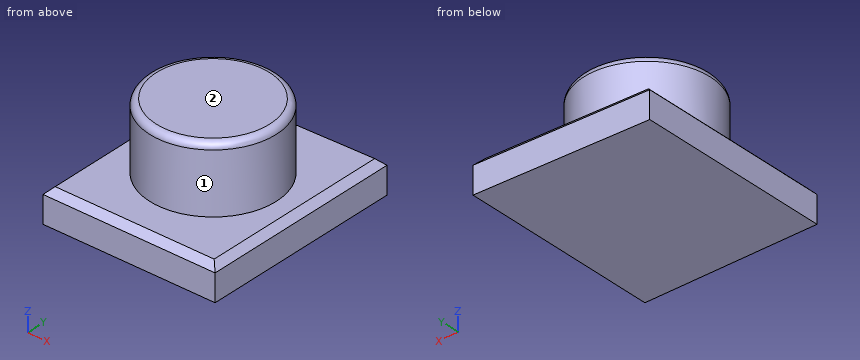
```python
from build123d import *

# Parameters (mm, degrees)
F1_DEPTH = 25.4
F2_R     = 48.0357441032
F3_DEPTH = 50.8
F4_R     = 5
F5_SIZE  = 5


# Not quite as in the source:
# - the program builds the solid bodies; features that only make, move or delete a surface that nothing else refers to are left out


with BuildPart() as f1:
    # F0 (on Top) → F1 (new body)
    with BuildSketch(Plane.XY):
        Polygon((118.1704625487, 0), (-12.6199126244, -4.1209459305), (-12.6199126244, -153.0908346176), (118.1704625487, -153.0908346176), align=None)
    extrude(amount=F1_DEPTH)

    # F2 (on face) → F3 (join)
    with BuildSketch(Plane.XY.offset(25.4)):
        with Locations((51.9535280764, -77.3641169071)):
            Circle(F2_R)
    extrude(amount=F3_DEPTH)

    # F4
    f4_edges = [f1.edges().sort_by_distance(p)[0] for p in [
        (3.917784, -77.364117, 76.2),
    ]]
    fillet(f4_edges, radius=F4_R)

    # F5
    f5_edges = [f1.edges().sort_by_distance(p)[0] for p in [
        (118.170463, -76.545417, 25.4),
        (52.775275, -2.060473, 25.4),
        (-12.619913, -78.60589, 25.4),
        (52.775275, -153.090835, 25.4),
    ]]
    chamfer(f5_edges, length=F5_SIZE)


solid = f1.part
```
Verification items for the finished model (mm, model axes). Face numbers are marked on the shaded views. A direction names the side the tool comes from. Round coordinates to 2 decimals unless told otherwise and drop trailing zeros. Write each loop counter-clockwise with the first axis right and the second up, starting at its lowest first coordinate (ties: lowest second). Pieces come first, ordered by that corner, then holes. Notation, with made-up numbers: (-26, 63) -> (9, 63) arc R19 ccw to (9, 94) -> close; hole circle Ø11 at (63, 21). An arc over 180 degrees is marked (long way). Write each question's results on one line, items separated by ' | '.
Q1. Sectioned sample at A-A, the plane y = -140. Record the boundary of the cut face in (x, z), and give its area (3 significant figures).
Derived:
outline: (-12.62, 0) -> (118.17, 0) -> (118.17, 20.4) -> (113.17, 25.4) -> (-7.62, 25.4) -> (-12.62, 20.4) -> close | area: 3,300 mm²
Q2. Access from +Z, -Z, +X, -X, +Y, -Y to the whole of each face (thin tool, end or side, straight path). Record for the marked faces 1 and 2.
Derived:
face 1: +Z | face 2: +Z, +X, -X, +Y, -Y
Q3. Sectioned sample at C-C, the plane z = 40. Record the boundary of the cut face in (x, y), and give its area (3 significant figures).
Derived:
outline: circle Ø96.07 at (51.95, -77.36) | area: 7,250 mm²
Q4. Go/stop test with flat-tipped pins: pin 1 Ø1.5 at (y, z) = (-110, 32.5) entering from -X; pin 2 Ø10 at (x, z) = (52.5, 10) entering from +Y; pin 3 Ø6 at (y, z) = (-101.5, 55) entering from -X. Record where each tip stops, or that it passes through.
Derived:
pin 1: stops at x = 16.03 | pin 2: stops at y = -1.91 | pin 3: stops at x = 8.82
Q5. Thickness scan on probe 1 along Z at (x, y) = (-4, -60.5); probe 2 along X at (y, z) = (-42.5, 25.5); probe 3 along Y at (x, z) = (89, 7). Record the ranges inside material, lowest first.
Derived:
probe 1: z = 0 to 25.4 | probe 2: x = 18.91 to 85 | probe 3: y = -153.09 to -0.92
Q6. Sectioned sample at B-B, the plane x = 103. Record the boundary of the cut face in (y, z).
Derived:
outline: (-153.09, 0) -> (-0.48, 0) -> (-0.48, 20.4) -> (-5.48, 25.4) -> (-148.09, 25.4) -> (-153.09, 20.4) -> close
